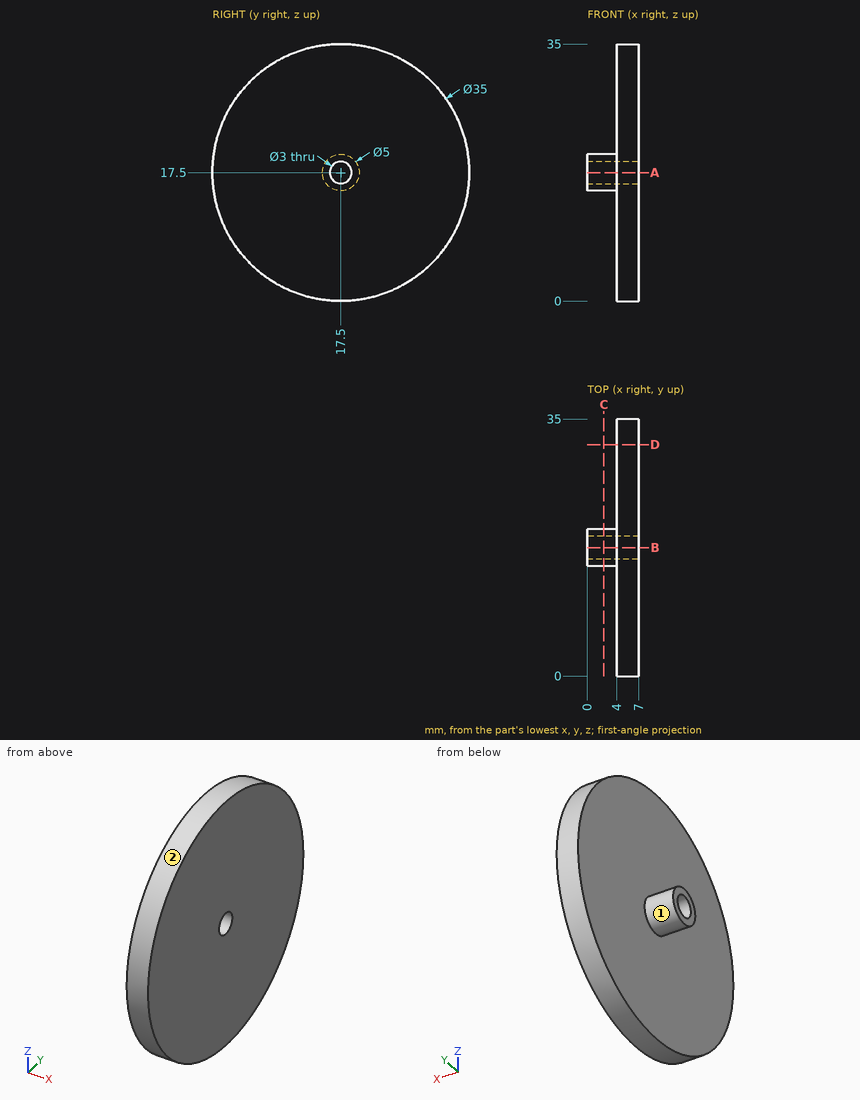
Part print with two shaded views. Sizes in mm from the minimum x, y, z corner. A direction names the side the tool comes from. Coordinates: 2 decimals unless noted, no trailing zeros. Write each loop counter-clockwise with the first axis right and the second up, starting at its lowest first coordinate (ties: lowest second). Pieces come first, ordered by that corner, then holes. Notation, with made-up numbers: M 59,74.25 L 80,74.25 A19 cw 80,80.25 Z; hole C -24,10 d6. An arc over 180 degrees is marked long. Return JSON: item names as keys, results as strings.
Item 1: Slice it at C-C, the plane x = 2.25. Write the cut outline in (y, z).
Findings below:
{"outline": "C 17.5,17.5 d5; hole C 17.5,17.5 d3"}
Item 2: Which spindle directions (+Z, -Z, +X, -X, +Y, -Y) get a long thin tool onto all of the face, cutting with end or side? Do the marked faces 1 and 2. Say none if no direction does.
Findings below:
{"face 1": "-X", "face 2": "+X, -X"}
Item 3: Slice it at D-D, the plane y = 31.5. Write the cut outline in (x, z).
Findings below:
{"outline": "M 4,7 L 7,7 L 7,28 L 4,28 Z"}
Item 4: Drop flat-ended pins along their axis: pin 1 Ø8 at (y, z) = (4, 25) entering from -X; pin 2 Ø5 at (y, z) = (17.5, 17.5) entering from -X; pin 3 Ø1 at (x, z) = (6.5, 31) entering from -Y. Give the stop position or say it passes through.
Findings below:
{"pin 1": "stops at x = 4", "pin 2": "stops at x = 0", "pin 3": "stops at y = 5.78"}
Item 5: Slice it at A-A, the plane z = 17.5. Write the cut outline in (x, y).
Findings below:
{"outline": "M 0,15 L 4,15 L 4,0 L 7,0 L 7,16 L 0,16 Z; M 0,19 L 7,19 L 7,35 L 4,35 L 4,20 L 0,20 Z"}
Item 6: Probe line 1 (Z direction, x = 2.5, y = 17.5); line 2 (X direction, y = 30.5, z = 29); line 3 (Z direction, x = 5.5, y = 17.5). List the from-to ranges inside material, lowest first. Write a range as from..to.
Findings below:
{"line 1": "z = 15..16, 19..20", "line 2": "x = 4..7", "line 3": "z = 0..16, 19..35"}
